Autodesk Inventor part; units mm, degrees
ref_plane "YZ Plane" through (0, 0, 0) normal (1, 0, 0) x (0, 1, 0)
ref_plane "XZ Plane" through (0, 0, 0) normal (0, 1, 0) x (-1, 0, 0)
ref_plane "XY Plane" through (0, 0, 0) normal (0, 0, 1) x (1, 0, 0)
sketch "Sketch1" plane through (0, 0, 0) normal (0, 0, 1) x (1, 0, 0)
  line L0 (0, 0) -> (25.4, 0)
  line L1 (25.4, 0) -> (25.4, 25.4)
  line L2 (25.4, 25.4) -> (0, 25.4)
  line L3 (0, 25.4) -> (0, 0)
  line L4 (1.5875, 23.8125) -> (23.8125, 23.8125)
  line L5 (23.8125, 23.8125) -> (23.8125, 1.5875)
  line L6 (23.8125, 1.5875) -> (1.5875, 1.5875)
  line L7 (1.5875, 1.5875) -> (1.5875, 23.8125)
  dimension "d0" = 25.4
  dimension "d1" = 25.4
  dimension "d2" = 1.5875
extrude "Extrusion1" add sketch "Sketch1" against normal blind 152.4
sketch "Sketch3" plane through (0, 0, 0) normal (0, -1, 0) x (1, 0, 0)
  line L0 (0, -152.4) -> (25.4, -152.4)
  line L1 (0, 0) -> (25.4, 0)
  line L2 (25.4, 0) -> (25.4, -152.4)
  point P0 (12.7, -12.7)
  point P1 (12.7, -139.7)
  point P2 (12.7, -50.8)
  dimension "d7" = 12.7
  dimension "d8" = 12.7
  dimension "d23" = 38.1
  dimension "d24" = 12.7
hole "Hole2" at (12.7, 0, -12.7) at (12.7, 0, -139.7) at (12.7, 0, -50.8) direction (0, 1, 0) diameter 6.35 depth 25.4 tip angle 118
properties part number "tube_f_l_out_wheel"
Build history of the part. All positions in model axes, mm. A direction names the side the tool comes from. Coordinates: 2 decimals unless noted, no trailing zeros. Order: outer loops, then holes, each group sorted by start corner. A loop starts at its lowest first (then second) coordinate and runs counter-clockwise, first axis right, second up. Notation, with made-up numbers: (57, 47) -> (84, 47) arc R25 ccw to (84, 83) -> close; hole circle Ø10 at (70.5, 22). An arc over 180 degrees is marked (long way). Answer in a Markdown table with one row per item. Add a question column.
Q1. Wall check: line 1 along Z through (x, y) = (12.7, 24.35) (3 decimals); line 2 along Y through (x, z) = (12.5, -92); line 3 along X through (y, z) = (24.25, -12.7) (3 decimals). Give the ranges that are in metal, low to high. Write a range as [from, to].
Q2. Mould opens along Z. For faces 3 (the face through (13.92, 24.62, -53.73)), 4 (the face through (13, 23.812, -75)), 5 (the face through (1, 13, -152.4)) say: +Z half, -Z half, draft (parallel to the pull), parting line (faces both ways), or undercut.
Q3. Band-saw the part on A-A, the plane x = 6.25. List the corners of the cut face in (y, z), then the cut area to 3 significant figures.
Q4. Band-saw the part on D-D, the plane x = 12.7. Give the number of separate pieces and of enclosed holes in the cut face, then the cut area to 3 significant figures.
Q5. Band-saw the part on B-B, the plane z = -19. List the corners of the cut face in (x, y).
Q6. Which spindle directions (+Z, -Z, +X, -X, +Y, -Y) get a long thin tool onto all of the face, cutting with end or side? Do faces 1 (the face through (25.4, 13, -75)), 2 (the face through (13, 1.588, -75)). Say none if no direction does.
Answers follow:
| question | item | result |
|---|---|---|
| 1 | line 1 | [-152.4, -142.875], [-136.525, -53.975], [-47.625, -15.875], [-9.525, 0] |
| 1 | line 2 | [0, 1.59], [23.81, 25.4] |
| 1 | line 3 | [0, 9.525], [15.875, 25.4] |
| 2 | face 3 | undercut |
| 2 | face 4 | draft |
| 2 | face 5 | -Z half |
| 3 | outline | (0, -152.4) -> (1.59, -152.4) -> (1.59, 0) -> (0, 0) -> close; (23.81, -152.4) -> (25.4, -152.4) -> (25.4, 0) -> (23.81, 0) -> close |
| 3 | area | 484 mm^2 |
| 4 | separate pieces | 8 |
| 4 | enclosed holes | 0 |
| 4 | area | 423 mm^2 |
| 5 | outline | (0, 0) -> (25.4, 0) -> (25.4, 25.4) -> (0, 25.4) -> close; hole (1.59, 1.59) -> (23.81, 1.59) -> (23.81, 23.81) -> (1.59, 23.81) -> close |
| 6 | face 1 | +Z, -Z, +X, +Y, -Y |
| 6 | face 2 | +Z, -Z |
